Work out the finished part from the listing and answer in its coordinate system (mm). A direction names the side the tool comes from. Give positions to 0.01 mm unless a question says otherwise; leave off trailing zeros. Loops run counter-clockwise (first coordinate to the right, second up) from the corner with the lowest first, then second, coordinate; pieces in that order, holes last. Notation, with made-up numbers: M -10.75,47 L 5.25,47 A15 ccw 5.25,74 Z; hole C 16,41.5 d6. An arc over 180 degrees is marked long. Answer in a Markdown table with one row per item. Add a question column.
from build123d import *

# Parameters (mm, degrees)
SKETCH_1_W      = 5
SKETCH_1_H      = 10
EXTRUDE_1_DEPTH = 70
SKETCH_2_W      = 5
SKETCH_2_H      = 10
EXTRUDE_2_DEPTH = 5


with BuildPart() as part:
    # 草图1 → 凸台-拉伸1 (new body)
    with BuildSketch(Plane(origin=(0, 0, 0), x_dir=(1, 0, 0), z_dir=(0, 1, 0))):
        with Locations((2.5, 5)):
            Rectangle(SKETCH_1_W, SKETCH_1_H)
    extrude(amount=EXTRUDE_1_DEPTH)

    # 草图2 → 凸台-拉伸2 (add)
    with BuildSketch(Plane(origin=(0, 70, 0), x_dir=(1, 0, 0), z_dir=(0, 1, 0))):
        with Locations((2.5, 15)):
            Rectangle(SKETCH_2_W, SKETCH_2_H)
        with Locations((2.5, 5)):
            Rectangle(SKETCH_2_W, SKETCH_2_H)
        with Locations((2.5, -5)):
            Rectangle(SKETCH_2_W, SKETCH_2_H)
    extrude(amount=EXTRUDE_2_DEPTH)


solid = part.part
(1) Section A-A, the plane x = 0.9 is taken. Determine the outline of the cut face in (y, z).
(2) Section B-B, the plane y = 39 is taken. Determine the outline of the cut face in (x, z), and give its area (3 significant figures).
(3) Consider line 1 along Z through (x, y) = (4.1, 53); line 2 along Y through (x, z) = (0.4, 4). Determine where each line is inside the solid, lowest interval first. Write a range as from..to.
(4) Which of the six approach directions +Z, -Z, +X, -X, +Y, -Y give full straight-line access (tool end or side, diameter ignored) to faces 1 (the face through (2, 35, -10)), 2 (the face through (2, 72, -20)), 3 (the face through (2, 70, 5))?
(5) Each of these flat-tipped pins is pushed along its axis until it touches: P1, Ø1.5, axis at x = 1.5, z = -13, coming from the -Y side; P2, Ø2.5, axis at x = 2.5, y = 26, coming from the +Z side. Where does it stop, or does it pass through?
(6) Section C-C, the plane z = -16 is taken. Determine the outline of the cut face in (x, y), and give its area (3 significant figures).
Numbers:
| question | item | result |
|---|---|---|
| 1 | outline | M 0,-10 L 70,-10 L 70,-20 L 75,-20 L 75,10 L 70,10 L 70,0 L 0,0 Z |
| 2 | outline | M 0,-10 L 5,-10 L 5,0 L 0,0 Z |
| 2 | area | 50.0 mm² |
| 3 | line 1 | z = -10..0 |
| 3 | line 2 | y = 70..75 |
| 4 | face 1 | -Z, +X, -X, -Y |
| 4 | face 2 | -Z, +X, -X, +Y, -Y |
| 4 | face 3 | +Z, +X, -X, -Y |
| 5 | P1 | stops at y = 70 |
| 5 | P2 | stops at z = 0 |
| 6 | outline | M 0,70 L 5,70 L 5,75 L 0,75 Z |
| 6 | area | 25.0 mm² |
